Verification items for the finished model (mm, model axes). Face numbers are marked on the shaded views. A direction names the side the tool comes from. Give positions to 0.01 mm unless a question says otherwise; leave off trailing zeros. Loops run counter-clockwise (first coordinate to the right, second up) from the corner with the lowest first, then second, coordinate; pieces in that order, holes last. Notation, with made-up numbers: (-15.75, 15.5) - (11.25, 15.5) arc R15 cw to (11.25, 34.5) - close; hole circle Ø9 at (86.25, 73). An arc over 180 degrees is marked (long way). One line per question, with ' | ' between items. Start each with the question number.
1. Depth check by flat-ended pin: pin 1 Ø11.5 at (y, z) = (-6.5, 95.5) entering from -X; pin 2 Ø3 at (y, z) = (2.5, 36) entering from +X; pin 3 Ø1.5 at (x, z) = (-27.5, 41.5) entering from +Y; pin 4 Ø22.5 at (y, z) = (0, 89.15) entering from -X. Enter the tip coordinate at first touch or a pass-through.
2. Section check B-B, the plane y = 0. Enter the section's corners in (x, z).
3. Tool access check on the marked faces 4, 5, 6, 7 and 8. Record the directions out of +Z, -Z, +X, -X, +Y, -Y that give a thin tool (end or side, any length) a straight path to the whole face; none if there is none.
4. Section check D-D, the plane x = -6. Enter the section's corners in (y, z), then the cut area to 3 significant figures.
5. Thickness scan on line 1 along Y through (x, z) = (-7.8, 89.15); line 2 along X through (y, z) = (-16, 69); line 3 along Z through (x, y) = (0, -0.5). Record the ranges inside material, lowest first. Write a range as from..to.
6. Mould release check, pull along X, two halves, no side actions. Record for the marked faces 1, 2 and 3: +X half, -X half, draft (parallel to the pull), parting line (faces both ways), or undercut.
7. Section check C-C, the plane z = 39. Enter the section's corners in (x, y) (3 decimals).
8. Section check A-A, the plane z = 89.15. Enter the section's corners in (x, y).
Autodesk Inventor part; units mm, degrees
ref_plane "YZ Plane" through (0, 0, 0) normal (1, 0, 0) x (0, 1, 0)
ref_plane "XZ Plane" through (0, 0, 0) normal (0, 1, 0) x (-1, 0, 0)
ref_plane "XY Plane" through (0, 0, 0) normal (0, 0, 1) x (1, 0, 0)
sketch "Sketch1" plane through (0, 0, 0) normal (0, 0, 1) x (1, 0, 0)
  circle A0 centre (0, 0) radius 11.25
  circle A1 centre (0, 0) radius 35.025
  circle A2 centre (0, 0) radius 37.030393
  arc A3 (-32.79294, -17.200962) -> (-31.29294, -19.799038) centre (0, 0) ccw
  line L0 (-32.79294, -17.200962) -> (-31.05471, -16.197395)
  line L1 (-32.79294, -17.200962) -> (-31.05471, -16.197395)
  line L2 (-29.55471, -18.795471) -> (-31.29294, -19.799038)
  line L3 (-31.29294, -19.799038) -> (-29.55471, -18.795471)
  line L4 (-16.197395, -31.05471) -> (-17.200962, -32.79294)
  line L5 (-17.200962, -32.79294) -> (-16.197395, -31.05471)
  arc A4 (-19.799038, -31.29294) -> (-17.200962, -32.79294) centre (0, 0) ccw
  line L6 (-19.799038, -31.29294) -> (-18.795471, -29.55471)
  line L7 (-19.799038, -31.29294) -> (-18.795471, -29.55471)
  arc A5 (17.200962, -32.79294) -> (19.799038, -31.29294) centre (0, 0) ccw
  line L8 (17.200962, -32.79294) -> (16.197395, -31.05471)
  line L9 (17.200962, -32.79294) -> (16.197395, -31.05471)
  line L10 (18.795471, -29.55471) -> (19.799038, -31.29294)
  line L11 (19.799038, -31.29294) -> (18.795471, -29.55471)
  arc A6 (31.29294, -19.799038) -> (32.79294, -17.200962) centre (0, 0) ccw
  line L12 (31.29294, -19.799038) -> (29.55471, -18.795471)
  line L13 (31.05471, -16.197395) -> (32.79294, -17.200962)
  line L14 (32.79294, -17.200962) -> (31.05471, -16.197395)
  line L15 (32.79294, 17.200962) -> (31.05471, 16.197395)
  line L16 (32.79294, 17.200962) -> (31.05471, 16.197395)
  arc A7 (32.79294, 17.200962) -> (31.29294, 19.799038) centre (0, 0) ccw
  line L17 (29.55471, 18.795471) -> (31.29294, 19.799038)
  line L18 (31.29294, 19.799038) -> (29.55471, 18.795471)
  line L19 (16.197395, 31.05471) -> (17.200962, 32.79294)
  line L20 (17.200962, 32.79294) -> (16.197395, 31.05471)
  line L21 (19.799038, 31.29294) -> (18.795471, 29.55471)
  line L22 (19.799038, 31.29294) -> (18.795471, 29.55471)
  line L23 (-17.200962, 32.79294) -> (-16.197395, 31.05471)
  line L24 (-17.200962, 32.79294) -> (-16.197395, 31.05471)
  line L25 (-18.795471, 29.55471) -> (-19.799038, 31.29294)
  line L26 (-19.799038, 31.29294) -> (-18.795471, 29.55471)
  arc A8 (-31.29294, 19.799038) -> (-32.79294, 17.200962) centre (0, 0) ccw
  line L27 (-31.29294, 19.799038) -> (-29.55471, 18.795471)
  line L28 (-31.29294, 19.799038) -> (-29.55471, 18.795471)
  line L29 (-31.05471, 16.197395) -> (-32.79294, 17.200962)
  line L30 (-32.79294, 17.200962) -> (-31.05471, 16.197395)
  arc A9 (-34.800207, -3.961848) -> (-34.800207, 3.961848) centre (-31.75, 0) ccw
  circle A10 centre (-31.75, 0) radius 5
  arc A11 (-3.961848, 34.800207) -> (3.961848, 34.800207) centre (0, 31.75) ccw
  circle A12 centre (0, 31.75) radius 5
  circle A13 centre (31.75, 0) radius 5
  circle A14 centre (31.75, 0) radius 5
  arc A15 (-3.961848, -34.800207) -> (3.961848, -34.800207) centre (0, -31.75) ccw
  circle A16 centre (0, -31.75) radius 5
  circle A17 centre (0, 31.75) radius 4.75
  circle A18 centre (-31.75, 0) radius 4.75
  circle A19 centre (0, -31.75) radius 4.75
  circle A20 centre (31.75, 0) radius 4.75
  circle A21 centre (0, 0) radius 34.775
  circle A22 centre (0, 0) radius 36.75
  point P0 (0, 0)
  point P1 (0, 49.75)
  point P2 (34.563789, -3.82689)
  point P3 (34.563789, 3.82689)
  point P4 (3.82689, 34.563789)
  point P5 (-3.82689, 34.563789)
  point P6 (-34.563789, 3.82689)
  point P7 (-34.563789, -3.82689)
  point P8 (-3.82689, -34.563789)
  point P9 (3.82689, -34.563789)
  dimension "d6" = 70.05
  dimension "d8" = 74.06079
  dimension "d0" = 10
  dimension "d1" = 0.25
  dimension "d4" = 360
  dimension "d7" = 0.25
  dimension "d9" = 73.5
sketch "Sketch1 outline for Extrusion1" plane through (0, 0, 0) normal (0, 0, 1) x (1, 0, 0)
  arc A0 (3.82689, -34.563789) -> (34.563789, -3.82689) centre (0, 0) ccw
  arc A1 (-3.82689, -34.563789) -> (3.82689, -34.563789) centre (0, -31.75) ccw
  arc A2 (-34.563789, -3.82689) -> (-3.82689, -34.563789) centre (0, 0) ccw
  arc A3 (-34.563789, 3.82689) -> (-34.563789, -3.82689) centre (-31.75, 0) ccw
  arc A4 (-3.82689, 34.563789) -> (-34.563789, 3.82689) centre (0, 0) ccw
  arc A5 (3.82689, 34.563789) -> (-3.82689, 34.563789) centre (0, 31.75) ccw
  arc A6 (34.563789, 3.82689) -> (3.82689, 34.563789) centre (0, 0) ccw
  arc A7 (34.563789, -3.82689) -> (34.563789, 3.82689) centre (31.75, 0) ccw
extrude "Extrusion1" add sketch "Sketch1 outline for Extrusion1" along normal blind 68.9
sketch "Skizze4" plane through (0, 0, 68.9) normal (0, 0, 1) x (1, 0, 0)
  line L0 (-9.75, 21.75) -> (9.75, 21.75) construction
  line L1 (9.75, 21.75) -> (9.75, -21.75) construction
  line L2 (9.75, -21.75) -> (-9.75, -21.75) construction
  line L3 (-9.75, -21.75) -> (-9.75, 21.75) construction
  line L4 (-9.75, 21.75) -> (9.75, -21.75) construction
  line L5 (9.75, 21.75) -> (-9.75, -21.75) construction
  line L6 (-9.75, 21.75) -> (-7.25, 21.75)
  line L7 (-7.25, 21.75) -> (-7.25, -21.75)
  line L8 (-7.25, -21.75) -> (-9.75, -21.75)
  line L9 (-9.75, -21.75) -> (-9.75, 21.75)
  line L10 (9.75, 21.75) -> (7.25, 21.75)
  line L11 (7.25, 21.75) -> (7.25, -21.75)
  line L12 (7.25, -21.75) -> (9.75, -21.75)
  line L13 (9.75, -21.75) -> (9.75, 21.75)
  line L14 (-7.25, -21.75) -> (8.25, -21.75)
  line L15 (8.25, -21.75) -> (8.25, -19.25)
  line L16 (8.25, -19.25) -> (-7.25, -19.25)
  line L17 (-7.25, -19.25) -> (-7.25, -21.75)
  line L18 (-7.25, 21.75) -> (8.25, 21.75)
  line L19 (8.25, 21.75) -> (8.25, 19.25)
  line L20 (8.25, 19.25) -> (-7.25, 19.25)
  line L21 (-7.25, 19.25) -> (-7.25, 21.75)
  point P0 (0, 0)
  point P1 (7.25, 19.25)
  point P2 (7.25, -19.25)
  dimension "d24" = 19.5
  dimension "d25" = 43.5
  dimension "d26" = 2.5
  dimension "d27" = 2.5
  dimension "d28" = 15.5
  dimension "d29" = 2.5
  dimension "d30" = 15.5
  dimension "d31" = 2.5
extrude "Extrusion4" add sketch "Skizze4" along normal blind 40.5 contours L6 L7 L8 L9 | L18 L11 L20 L7 | L10 L19 L20 L11 | L7 L16 L11 L14 | L20 L19 L10 L13 L12 L15 L16 L11 | L11 L16 L15 L12
sketch "Skizze5" plane through (9.75, -21.75, 68.9) normal (1, 0, 0) x (0, 0, -1)
  line L0 (-40.5, 43.5) -> (-40.5, 0) construction
  line L1 (0, 0) -> (-40.5, 0) construction
  line L2 (-40.5, 43.5) -> (0, 0) construction
  line L3 (0, 43.5) -> (-40.5, 43.5) construction
  line L4 (0, 43.5) -> (-40.5, 0) construction
  circle A0 centre (-20.25, 21.75) radius 14
  point P0 (68.9, 21.75)
  dimension "d35" = 28
extrude "Extrusion5" cut sketch "Skizze5" against normal through all
properties part number "power_sensor_aperture_V1.1"
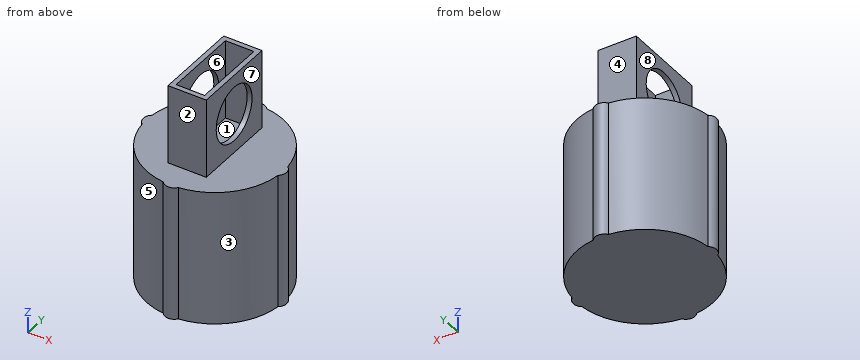
Results list:
1) pin 1: x = -9.75 | pin 2: x = 36.39 | pin 3: y = 22.22 | pin 4: through
2) outline: (-36.5, 0) - (36.5, 0) - (36.5, 68.9) - (9.75, 68.9) - (9.75, 75.15) - (7.25, 75.15) - (7.25, 68.9) - (-7.25, 68.9) - (-7.25, 75.15) - (-9.75, 75.15) - (-9.75, 68.9) - (-36.5, 68.9) - close; (-9.75, 103.15) - (-7.25, 103.15) - (-7.25, 109.4) - (-9.75, 109.4) - close; (7.25, 103.15) - (9.75, 103.15) - (9.75, 109.4) - (7.25, 109.4) - close
3) face 4: +Z, +X, -X, +Y | face 5: +Z, -Z, -X, -Y | face 6: +Z | face 7: +Z, +X, +Y, -Y | face 8: +Z, -X, +Y, -Y
4) outline: (-34.25, 0) - (34.25, 0) - (34.25, 68.9) - (21.75, 68.9) - (21.75, 109.4) - (19.25, 109.4) - (19.25, 68.9) - (-19.25, 68.9) - (-19.25, 109.4) - (-21.75, 109.4) - (-21.75, 68.9) - (-34.25, 68.9) - close | area: 4,920 mm²
5) line 1: -21.75..-14, 14..21.75 | line 2: -9.75..-7.25, 7.25..9.75 | line 3: 0..68.9
6) face 1: undercut | face 2: draft | face 3: +X half
7) outline: (-34.564, -3.827) arc R34.775 ccw to (-3.827, -34.564) arc R4.75 ccw to (3.827, -34.564) arc R34.775 ccw to (34.564, -3.827) arc R4.75 ccw to (34.564, 3.827) arc R34.775 ccw to (3.827, 34.564) arc R4.75 ccw to (-3.827, 34.564) arc R34.775 ccw to (-34.564, 3.827) arc R4.75 ccw to start
8) outline: (-9.75, -21.75) - (9.75, -21.75) - (9.75, -14) - (7.25, -14) - (7.25, -19.25) - (-7.25, -19.25) - (-7.25, -14) - (-9.75, -14) - close; (-9.75, 14) - (-7.25, 14) - (-7.25, 19.25) - (7.25, 19.25) - (7.25, 14) - (9.75, 14) - (9.75, 21.75) - (-9.75, 21.75) - close
